The model under review builds one solid part; all positions refer to its coordinate system, in mm. Give positions to 0.01 mm unless a question says otherwise; leave off trailing zeros. Write each loop counter-clockwise with the first axis right and the second up, starting at its lowest first coordinate (ties: lowest second). Pieces come first, ordered by that corner, then holes. Notation, with made-up numbers: (21, 55.25) - (71, 55.25) arc R17 cw to (71, 80.25) - close; hole circle Ø5 at (2, 25). An arc over 180 degrees is marked (long way). Write item = value, one per line.
Autodesk Inventor part; units mm, degrees
ref_plane "YZ Plane" through (0, 0, 0) normal (1, 0, 0) x (0, 1, 0)
ref_plane "XZ Plane" through (0, 0, 0) normal (0, 1, 0) x (-1, 0, 0)
ref_plane "XY Plane" through (0, 0, 0) normal (0, 0, 1) x (1, 0, 0)
sketch "Sketch1" plane through (0, 0, 0) normal (0, 0, 1) x (1, 0, 0)
  circle A0 centre (0, 0) radius 63.5 construction
  circle A1 centre (0, 0) radius 88.9 construction
  line L0 (0, 88.9) -> (-37.3244, 51.3726)
  line L1 (-37.3244, 51.3726) -> (-84.5489, 27.4716)
  line L2 (-84.5489, 27.4716) -> (-60.3921, -19.6226)
  line L3 (-60.3921, -19.6226) -> (-52.2541, -71.9216)
  line L4 (-52.2541, -71.9216) -> (0, -63.5)
  line L5 (52.2541, -71.9216) -> (0, -63.5)
  line L6 (60.3921, -19.6226) -> (52.2541, -71.9216)
  line L7 (60.3921, -19.6226) -> (84.5489, 27.4716)
  line L8 (84.5489, 27.4716) -> (37.3244, 51.3726)
  line L9 (37.3244, 51.3726) -> (0, 88.9)
  dimension "d0" = 127
  dimension "d1" = 177.8
  dimension "d4" = 360
  dimension "d8" = 360
extrude "Extrusion1" add sketch "Sketch1" along normal blind 3.175
sketch "Sketch2" plane through (0, 0, 3.175) normal (0, 0, 1) x (1, 0, 0)
  line L0 (37.3244, 51.3726) -> (0, 88.9)
  line L1 (84.5489, 27.4716) -> (37.3244, 51.3726)
  line L2 (60.3921, -19.6226) -> (84.5489, 27.4716)
  line L3 (52.2541, -71.9216) -> (60.3921, -19.6226)
  line L4 (0, -63.5) -> (52.2541, -71.9216)
  line L5 (-21.3489, 67.4349) -> (-19.0978, 65.1959)
  line L6 (-19.0978, 65.1959) -> (-13.7243, 70.5987)
  line L7 (-13.7243, 70.5987) -> (-15.9754, 72.8377)
  line L8 (-21.3489, 67.4349) -> (-15.9754, 72.8377)
  line L9 (0, 70.1363) -> (0, 60.325) construction
  line L10 (21.3489, 67.4349) -> (19.0978, 65.1959)
  line L11 (19.0978, 65.1959) -> (13.7243, 70.5987)
  line L12 (13.7243, 70.5987) -> (15.9754, 72.8377)
  line L13 (21.3489, 67.4349) -> (15.9754, 72.8377)
  line L14 (-64.3361, 37.7016) -> (-62.9023, 34.8688)
  line L15 (-62.9023, 34.8688) -> (-56.1035, 38.3097)
  line L16 (-56.1035, 38.3097) -> (-57.5372, 41.1426)
  line L17 (0, 0) -> (-84.5489, 27.4716) construction
  line L18 (-64.3361, 37.7016) -> (-57.5372, 41.1426)
  line L19 (-74.2094, 7.3145) -> (-71.3844, 8.7636)
  line L20 (-71.3844, 8.7636) -> (-67.9066, 1.9836)
  line L21 (-67.9066, 1.9836) -> (-70.7316, 0.5345)
  line L22 (-74.2094, 7.3145) -> (-70.7316, 0.5345)
  line L23 (-56.9089, -42.0074) -> (-55.7373, -49.5368)
  line L24 (-55.7373, -49.5368) -> (-52.6, -49.0486)
  line L25 (-52.6, -49.0486) -> (-53.7717, -41.5192)
  line L26 (-53.7717, -41.5192) -> (-56.9089, -42.0074)
  line L27 (-52.2541, -71.9216) -> (0, 0) construction
  line L28 (-22.3656, -67.1046) -> (-29.8885, -68.317)
  line L29 (-29.8885, -68.317) -> (-30.3937, -65.1825)
  line L30 (-30.3937, -65.1825) -> (-22.8708, -63.97)
  line L31 (-22.8708, -63.97) -> (-22.3656, -67.1046)
  line L32 (64.3361, 37.7016) -> (62.9023, 34.8688)
  line L33 (62.9023, 34.8688) -> (56.1035, 38.3097)
  line L34 (56.1035, 38.3097) -> (57.5372, 41.1426)
  line L35 (64.3361, 37.7016) -> (57.5372, 41.1426)
  line L36 (71.3844, 8.7636) -> (67.9066, 1.9836)
  line L37 (67.9066, 1.9836) -> (70.7316, 0.5345)
  line L38 (74.2094, 7.3145) -> (70.7316, 0.5345)
  line L39 (74.2094, 7.3145) -> (71.3844, 8.7636)
  line L40 (56.9089, -42.0074) -> (55.7373, -49.5368)
  line L41 (55.7373, -49.5368) -> (52.6, -49.0486)
  line L42 (52.6, -49.0486) -> (53.7717, -41.5192)
  line L43 (53.7717, -41.5192) -> (56.9089, -42.0074)
  line L44 (29.8885, -68.317) -> (30.3937, -65.1825)
  line L45 (22.3656, -67.1046) -> (29.8885, -68.317)
  line L46 (30.3937, -65.1825) -> (22.8708, -63.97)
  line L47 (22.8708, -63.97) -> (22.3656, -67.1046)
  line L48 (-37.3244, 51.3726) -> (-84.5489, 27.4716)
  line L49 (0, 88.9) -> (-37.3244, 51.3726)
  line L50 (-84.5489, 27.4716) -> (-60.3921, -19.6226)
  line L51 (-60.3921, -19.6226) -> (-52.2541, -71.9216)
  line L52 (-52.2541, -71.9216) -> (0, -63.5)
  point P0 (-18.6622, 70.1363)
  point P1 (18.6622, 70.1363)
  point P2 (60.9366, 39.4221)
  point P3 (72.4705, 3.9245)
  point P4 (56.3231, -45.7721)
  point P5 (-56.3231, -45.7721)
  point P6 (-72.4705, 3.9245)
  point P7 (-60.9366, 39.4221)
  point P8 (-26.1271, -67.7108)
  point P9 (26.1271, -67.7108)
  dimension "d12" = 3.81
  dimension "d13" = 3.81
  dimension "d14" = 3.175
  dimension "d15" = 3.81
  dimension "d16" = 7.62
  dimension "d18" = 3.81
extrude "Extrusion2" cut sketch "Sketch2" against normal blind 25.4 contours L10 L11 L12 L0 | L1 L32 L33 L34 | L7 L6 L5 L8 | L2 L37 L36 L39 | L16 L15 L14 L18 | L3 L41 L42 L43 | L19 L20 L21 L22 | L4 L47 L46 L44 | L26 L25 L24 L23 | L28 L29 L30 L31
sketch "Sketch3" plane through (0, 0, 0) normal (1, 0, 0) x (0, 1, 0)
  line L0 (0, 3.175) -> (0, 185.8962) construction
  line L1 (88.9, 0) -> (88.9, 3.175)
  point P0 (0, 0)
  point P1 (0.5345, 3.175)
  dimension "d22" = 88.9
  dimension "d23" = 182.7212
sketch "Sketch4" plane through (0, 0, 3.175) normal (0, 0, 1) x (1, 0, 0)
  line L0 (-39.8185, 34.4573) -> (0, 74.4925)
  line L1 (0, 74.4925) -> (39.8185, 34.4573)
  line L2 (39.8185, 34.4573) -> (39.8039, 29.0692)
  line L3 (39.8039, 29.0692) -> (0, 69.0896)
  line L4 (0, 69.0896) -> (-39.8039, 29.0692)
  line L5 (-39.8039, 29.0692) -> (-39.8185, 34.4573)
  line L6 (-21.3489, 67.4349) -> (-37.3244, 51.3726)
  line L7 (37.3244, 51.3726) -> (21.3489, 67.4349)
  line L8 (-50.5051, -17.0826) -> (-43.7856, -60.2657)
  line L9 (-43.7856, -60.2657) -> (0, -53.2089)
  line L10 (0, -53.2089) -> (43.7856, -60.2657)
  line L11 (43.7856, -60.2657) -> (50.5051, -17.0826)
  line L12 (50.5051, -17.0826) -> (46.1546, -20.2615)
  line L13 (46.1546, -20.2615) -> (40.6099, -55.8947)
  line L14 (40.6099, -55.8947) -> (0, -49.3497)
  line L15 (0, -49.3497) -> (-40.6099, -55.8947)
  line L16 (-40.6099, -55.8947) -> (-46.1546, -20.2615)
  line L17 (-46.1546, -20.2615) -> (-50.5051, -17.0826)
  line L18 (-55.7373, -49.5368) -> (-52.2541, -71.9216)
  line L19 (52.2541, -71.9216) -> (55.7373, -49.5368)
  line L20 (29.8885, -68.317) -> (52.2541, -71.9216)
  line L21 (0, -63.5) -> (22.3656, -67.1046)
  line L22 (-22.3656, -67.1046) -> (0, -63.5)
  line L23 (-52.2541, -71.9216) -> (-29.8885, -68.317)
  line L24 (-37.3244, 51.3726) -> (-57.5372, 41.1426)
  point P0 (0, 0)
  point P1 (-60.3921, -19.6226)
  point P2 (60.3921, -19.6226)
  dimension "d24" = 3.81
  dimension "d26" = 10.16
  dimension "d27" = 10.16
  dimension "d29" = 3.81
  dimension "d30" = 2.54
  dimension "d32" = 2.54
  dimension "d33" = 3.81
  dimension "d34" = 3.81
  dimension "d35" = 3.81
  dimension "d36" = 3.81
  dimension "d37" = 10.16
  dimension "d38" = 10.16
  dimension "d39" = 10.16
  dimension "d40" = 10.16
  dimension "d44" = 45
  dimension "d45" = 45
  dimension "d46" = 45
  dimension "d47" = 45
  dimension "d48" = 2.54
  dimension "d50" = 2.54
extrude "Extrusion3" cut sketch "Sketch4" against normal blind 25.4
properties part number "Star Base" material "Wood (Birch)"
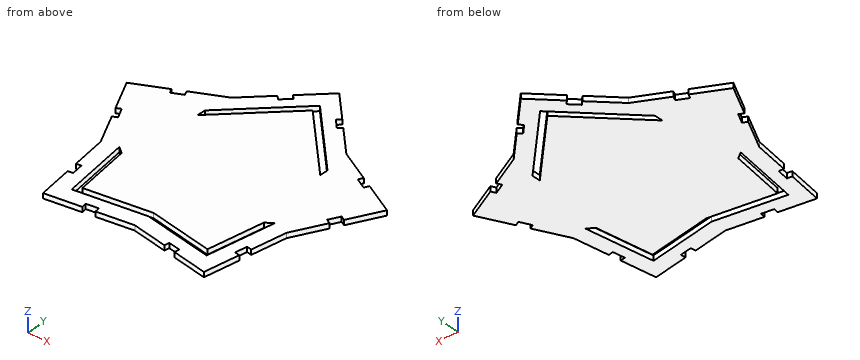
1. Take a section at B-B on y = -10.5. Give the boundary of the cut face in (x, z) (1 decimal), and give its area (3 significant figures).
Findings below:
outline = (-65.1, 0) - (65.1, 0) - (65.1, 3.2) - (-65.1, 3.2) - close
area = 413 mm²
2. Take a section at C-C on z = 2.55. Count the separate pieces of the cut face and the enclosed holes in it, and give its area (3 significant figures).
Findings below:
separate_pieces = 1
enclosed_holes = 2
area = 15,300 mm²
3. Take a section at A-A on x = -6.5. Give the boundary of the cut face in (y, z) (3 decimals), and give its area (3 significant figures).
Findings below:
outline = (-64.548, 0) - (-54.256, 0) - (-54.256, 3.175) - (-64.548, 3.175) - close; (-50.397, 0) - (62.554, 0) - (62.554, 3.175) - (-50.397, 3.175) - close; (67.957, 0) - (82.365, 0) - (82.365, 3.175) - (67.957, 3.175) - close
area = 437 mm²
4. For line 1 (X direction, y = -32, z = 2.9); line 2 (X direction, y = -36, z = 2.9); line 3 (Y direction, x = -38.5, z = 0.5), list the stretches that pass through material, from the lowest coordinate up. Write a range as from..to.
Findings below:
line_1 = -58.47..-48.18, -44.33..44.33, 48.18..58.47
line_2 = -57.84..-47.56, -43.71..43.71, 47.56..57.84
line_3 = -69.7..-59.41, -55.55..30.38, 35.78..50.78
